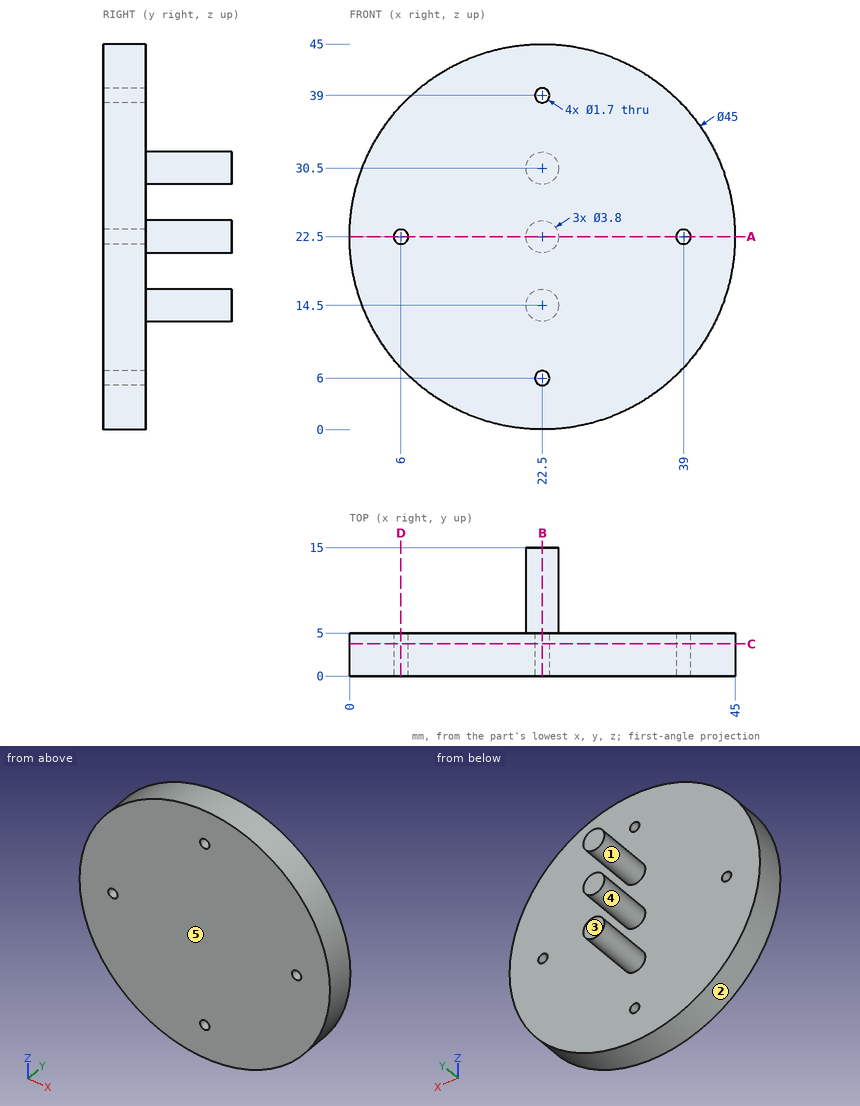
The drawing under review shows one solid part. Ordinate dimensions are in mm from its lowest x, y, z. A direction names the side the tool comes from. Round coordinates to 2 decimals unless told otherwise and drop trailing zeros. Loops run counter-clockwise (first coordinate to the right, second up) from the corner with the lowest first, then second, coordinate; pieces in that order, holes last. Notation, with made-up numbers: (60.25, 79.5) - (112.25, 79.5) arc R22 ccw to (112.25, 99.5) - close; hole circle Ø8 at (88.25, 57.25). An arc over 180 degrees is marked (long way). Put each result on its own line as item: value. Start each with the question number.
1. For the marked faces 4 and 5, list the 3-axis set-ups (+Z, -Z, +X, -X, +Y, -Y) from which the entire face can be reached by the end or side of a thin tool; tool diameter is ignored.
2. For probe 1 along Z at (x, y) = (22.5, 1.9); probe 2 along Z at (x, y) = (39, 1.1); probe 3 along Y at (x, z) = (10, 30), list the stretches that pass through material, from the lowest coordinate up. Write a range as [from, to].
3. Insertion check: P1, Ø5, axis at x = 19, y = 3, coming from the -Z side; P2, Ø2, axis at x = 26, y = 1.5, coming from the -Z side; P3, Ø10, axis at x = 13.5, z = 8.5, coming from the +Y side; P4, Ø1.4, axis at x = 22.5, z = 6, coming from the -Y side. Each pin has a flat end and moves straight along its axis. Give the tip position at first contact, or say it passes through.
4. Mouldability with a two-part tool opening along Z and no side actions: class the marked faces 1, 2 and 3 as +Z half, -Z half, draft (parallel to the pull), parting line (faces both ways), or undercut.
5. Consider section A-A on z = 22.5. State the section outline as (x, y) points.
6. Consider section C-C on y = 3.75. State the section outline as (x, z) points, plus the area to 3 significant figures.
7. Consider section D-D on x = 6. State the section outline as (y, z) points.
8. Consider section B-B on x = 22.5. State the section outline as (y, z) points.
Result sheet:
1. face 4: +Y
1. face 5: +Z, -Z, +X, -X, -Y
2. probe 1: [0, 5.15], [6.85, 38.15], [39.85, 45]
2. probe 2: [7.2, 21.65], [23.35, 37.8]
2. probe 3: [0, 5]
3. P1: z = 0.02
3. P2: z = 0.14
3. P3: y = 5
3. P4: through
4. face 1: undercut
4. face 2: parting line
4. face 3: draft
5. outline: (0, 0) - (5.15, 0) - (5.15, 5) - (0, 5) - close; (6.85, 0) - (38.15, 0) - (38.15, 5) - (24.4, 5) - (24.4, 15) - (20.6, 15) - (20.6, 5) - (6.85, 5) - close; (39.85, 0) - (45, 0) - (45, 5) - (39.85, 5) - close
6. outline: circle Ø45 at (22.5, 22.5); hole circle Ø1.7 at (6, 22.5); hole circle Ø1.7 at (22.5, 6); hole circle Ø1.7 at (22.5, 39); hole circle Ø1.7 at (39, 22.5)
6. area: 1,580 mm^2
7. outline: (0, 7.2) - (5, 7.2) - (5, 21.65) - (0, 21.65) - close; (0, 23.35) - (5, 23.35) - (5, 37.8) - (0, 37.8) - close
8. outline: (0, 0) - (5, 0) - (5, 5.15) - (0, 5.15) - close; (0, 6.85) - (5, 6.85) - (5, 12.6) - (15, 12.6) - (15, 16.4) - (5, 16.4) - (5, 20.6) - (15, 20.6) - (15, 24.4) - (5, 24.4) - (5, 28.6) - (15, 28.6) - (15, 32.4) - (5, 32.4) - (5, 38.15) - (0, 38.15) - close; (0, 39.85) - (5, 39.85) - (5, 45) - (0, 45) - close
